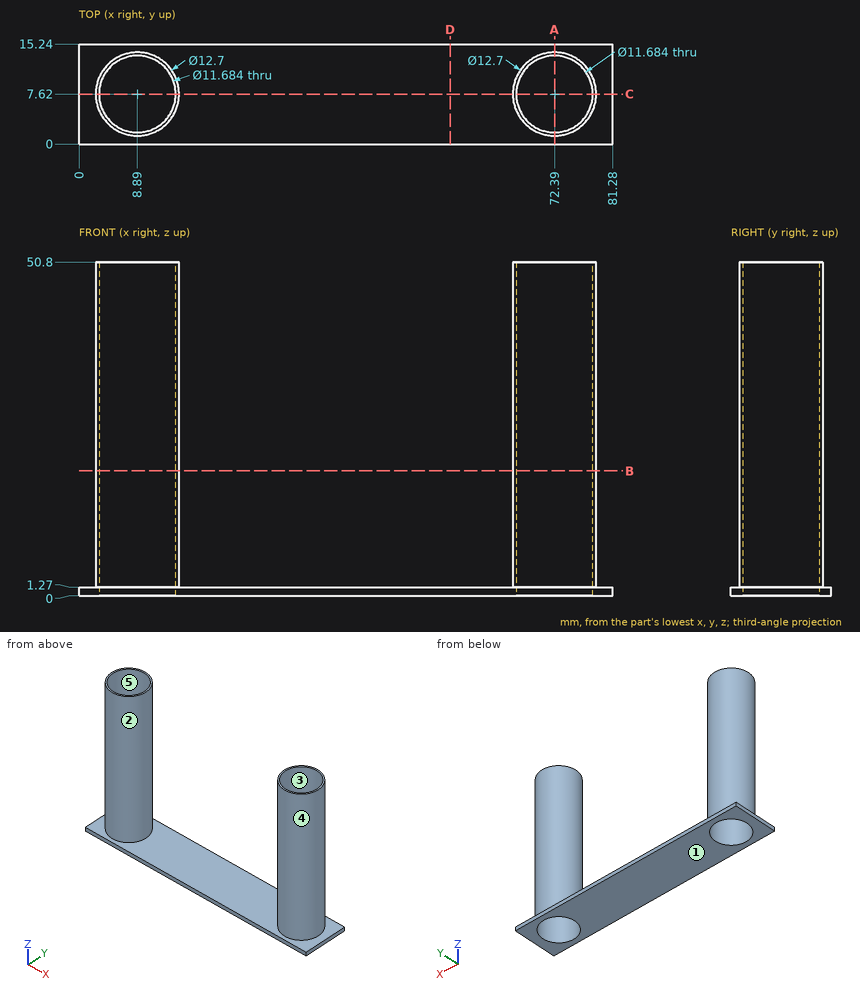
Here's the drawing with two shaded views (mm, measured from the low corner). I have some questions. A direction names the side the tool comes from. Round coordinates to 2 decimals unless told otherwise and drop trailing zeros. Loops run counter-clockwise (first coordinate to the right, second up) from the corner with the lowest first, then second, coordinate; pieces in that order, holes last. Notation, with made-up numbers: (11, -36.5) -> (16, -36.5) arc R17 cw to (16, -24.5) -> close; hole circle Ø11 at (60.5, -22.5). An arc over 180 degrees is marked (long way). Answer as CSV lines item,"result". Start each with the question number.
1. Imagine slicing it at C-C on y = 7.62. Write out the boundary of the cut face in (x, z), plus the area to 3 significant figures.
2. Imagine slicing it at D-D on x = 56.5. Write out the boundary of the cut face in (y, z).
3. If we mould it in two halves opening along Y, with no side actions, what happens to the marked faces 1, 2 and 3? For each: pulls with the +Y half, pulls with the -Y half, needs draft (parallel to the pull), parting line crosses it, or undercut.
4. I need wall thicknesses on probe 1 along X at (y, z) = (8, 6.5); probe 2 along Y at (x, z) = (8.89, 11); probe 3 along Y at (x, z) = (72, 26). Which ranges of each line are inside material? Lowest first, please. Write a range as from..to.
5. I'm going to push flat-ended pins straight in: P1, Ø1, axis at x = 10, z = 8, coming from the -Y side; P2, Ø6, axis at y = 9, z = 5.5, coming from the +X side; P3, Ø2, axis at x = 53.5, y = 2, coming from the +Z side; P4, Ø7, axis at x = 72.39, y = 7.62, coming from the +Z side. Where does each tip first touch, or does it pass through?
6. Imagine slicing it at B-B on z = 19. Write out the boundary of the cut face in (x, y), plus the area to 3 significant figures.
7. For the marked faces 4 and 5, which set-ups out of +Z, -Z, +X, -X, +Y, -Y let a thin tool reach every point of the face, with its end or its side?
8. Imagine slicing it at A-A on x = 72.39. Write out the boundary of the cut face in (y, z).
Solution:
1,outline,"(0, 0) -> (3.05, 0) -> (3.05, 50.8) -> (2.54, 50.8) -> (2.54, 1.27) -> (0, 1.27) -> close; (14.73, 0) -> (66.55, 0) -> (66.55, 50.8) -> (66.04, 50.8) -> (66.04, 1.27) -> (15.24, 1.27) -> (15.24, 50.8) -> (14.73, 50.8) -> close; (78.23, 0) -> (81.28, 0) -> (81.28, 1.27) -> (78.74, 1.27) -> (78.74, 50.8) -> (78.23, 50.8) -> close"
1,area,"174 mm²"
2,outline,"(0, 0) -> (15.24, 0) -> (15.24, 1.27) -> (0, 1.27) -> close"
3,face 1,"needs draft"
3,face 2,"parting line crosses it"
3,face 3,"undercut"
4,probe 1,"2.55..3.06, 14.72..15.23, 66.05..66.56, 78.22..78.73"
4,probe 2,"1.27..1.78, 13.46..13.97"
4,probe 3,"1.28..1.79, 13.45..13.96"
5,P1,"y = 1.3"
5,P2,"x = 78.74"
5,P3,"z = 1.27"
5,P4,"through"
6,outline,"circle Ø12.7 at (8.89, 7.62); circle Ø12.7 at (72.39, 7.62); hole circle Ø11.68 at (8.89, 7.62); hole circle Ø11.68 at (72.39, 7.62)"
6,area,"38.9 mm²"
7,face 4,"+Z"
7,face 5,"+Z, -Z"
8,outline,"(0, 0) -> (1.78, 0) -> (1.78, 50.8) -> (1.27, 50.8) -> (1.27, 1.27) -> (0, 1.27) -> close; (13.46, 0) -> (15.24, 0) -> (15.24, 1.27) -> (13.97, 1.27) -> (13.97, 50.8) -> (13.46, 50.8) -> close"
